Autodesk Inventor part; units mm, degrees
ref_plane "YZ Plane" through (0, 0, 0) normal (1, 0, 0) x (0, 1, 0)
ref_plane "XZ Plane" through (0, 0, 0) normal (0, 1, 0) x (-1, 0, 0)
ref_plane "XY Plane" through (0, 0, 0) normal (0, 0, 1) x (1, 0, 0)
sketch "Boceto1" plane through (0, 0, 0) normal (0, 1, 0) x (-1, 0, 0)
  line L0 (10, -10) -> (-10, -10)
  line L1 (-10, -10) -> (-10, 10)
  line L2 (-10, 10) -> (10, 10)
  line L3 (10, 10) -> (10, -10)
  line L4 (10, -10) -> (-10, 10) construction
  line L5 (-10, -10) -> (10, 10) construction
  point P0 (0, 0)
  dimension "d0" = 20
  dimension "d1" = 20
extrude "Extrusión1" add sketch "Boceto1" along normal blind 5
sketch "Boceto2" plane through (0, 0, 0) normal (0, -1, 0) x (1, 0, 0)
  circle A0 centre (0, 0) radius 3
  dimension "d4" = 6
extrude "Extrusión2" cut sketch "Boceto2" against normal blind 2.5
sketch "Boceto3" plane through (0, 5, 0) normal (0, 1, 0) x (1, 0, 0)
  line L0 (7.5, -7.5) -> (-7.5, -7.5)
  line L1 (-7.5, -7.5) -> (-7.5, 7.5)
  line L2 (-7.5, 7.5) -> (7.5, 7.5)
  line L3 (7.5, 7.5) -> (7.5, -7.5)
  line L4 (7.5, -7.5) -> (-7.5, 7.5) construction
  line L5 (-7.5, -7.5) -> (7.5, 7.5) construction
  circle A0 centre (-7.5, 7.5) radius 1.5
  circle A1 centre (7.5, 7.5) radius 1.5
  circle A2 centre (-7.5, -7.5) radius 1.5
  circle A3 centre (7.5, -7.5) radius 1.5
  point P0 (0, 0)
  dimension "d7" = 15
  dimension "d8" = 15
  dimension "d9" = 3
  dimension "d10" = 3
  dimension "d11" = 3
  dimension "d12" = 3
extrude "Extrusión3" cut sketch "Boceto3" against normal blind 5 contours A2 L1 L0 | L0 L1 A2 | A3 L3 L0 | L0 L3 A3 | A0 L2 L1 | L1 L2 A0 | A1 L2 L3 | L3 L2 A1
properties part number "engine_coupling" material "Plástico ABS"
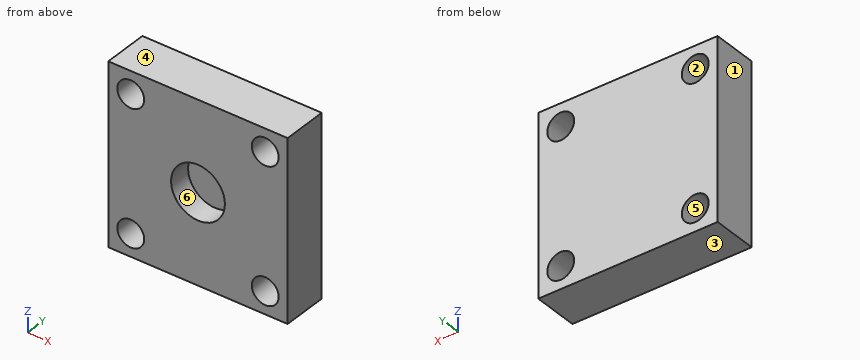
Work out the finished part from the listing and answer in its coordinate system (mm). Face numbers are marked on the shaded views. A direction names the side the tool comes from. Round coordinates to 2 decimals unless told otherwise and drop trailing zeros. Write each loop counter-clockwise with the first axis right and the second up, starting at its lowest first coordinate (ties: lowest second). Pieces come first, ordered by that corner, then holes.
1) Flat-ended cylindrical pins translate along their axes: P1, Ø1.8, axis at x = 0.5, z = 0, coming from the -Y side; P2, Ø3.5, axis at x = 7.5, z = -7.5, coming from the +Y side. Find the tip coordinate at first contact, or state that the pin passes through.
2) Consider probe 1 along X at (y, z) = (1.35, 7.5); probe 2 along X at (y, z) = (3.45, -8.75). Determine where each line is inside the solid, lowest interval first.
3) A cutting plane is placed at C-C on x = 7.5. Determine the outline of the cut face in (y, z), and give its area (3 significant figures).
4) Determine the mould class of the marked faces 1, 2, 3 and 4 for opening direction Z: pulls with the +Z half, pulls with the -Z half, needs draft (parallel to the pull), parting line crosses it, or undercut.
5) A cutting plane is placed at D-D on z = 0. Determine the outline of the cut face in (x, y).
6) A cutting plane is placed at B-B on y = 4.15. Determine the outline of the cut face in (x, z).
7) A cutting plane is placed at A-A on z = -7.5. Determine the outline of the cut face in (x, y), and give its area (3 significant figures).
8) Which of the six approach directions +Z, -Z, +X, -X, +Y, -Y give full straight-line access (tool end or side, diameter ignored) to the marked faces 5 and 6?
Entries:
1. P1: stops at y = 2.5
1. P2: stops at y = 5
2. probe 1: x = -10 to -9, -6 to 6, 9 to 10
2. probe 2: x = -10 to -8.33, -6.67 to 6.67, 8.33 to 10
3. outline: (0, -10) - (5, -10) - (5, -9) - (0, -9) - close; (0, -6) - (5, -6) - (5, 6) - (0, 6) - close; (0, 9) - (5, 9) - (5, 10) - (0, 10) - close
3. area: 70.0 mm2
4. face 1: needs draft
4. face 2: undercut
4. face 3: pulls with the -Z half
4. face 4: pulls with the +Z half
5. outline: (-10, 0) - (-3, 0) - (-3, 2.5) - (3, 2.5) - (3, 0) - (10, 0) - (10, 5) - (-10, 5) - close
6. outline: (-10, -10) - (10, -10) - (10, 10) - (-10, 10) - close; hole circle Ø3 at (-7.5, -7.5); hole circle Ø3 at (-7.5, 7.5); hole circle Ø3 at (7.5, -7.5); hole circle Ø3 at (7.5, 7.5)
7. outline: (-10, 0) - (-9, 0) - (-9, 5) - (-10, 5) - close; (-6, 0) - (6, 0) - (6, 5) - (-6, 5) - close; (9, 0) - (10, 0) - (10, 5) - (9, 5) - close
7. area: 70.0 mm2
8. face 5: +Y, -Y
8. face 6: -Y
